Check sheet for the drawn part. Datum: minimum x, y, z corner. Units: mm. A direction names the side the tool comes from. Coordinates: 2 decimals unless noted, no trailing zeros. Write each loop counter-clockwise with the first axis right and the second up, starting at its lowest first coordinate (ties: lowest second). Pieces come first, ordered by that corner, then holes. Notation, with made-up numbers: (-19.5, -20.75) -> (0.5, -20.75) arc R26 cw to (0.5, 15.25) -> close; hole circle Ø2 at (-39, -7.5). An arc over 180 degrees is marked (long way). Answer in a Markdown table with one row per item. Add a question column.
Q1. Thickness scan on line 1 (Z direction, x = 10, y = 63.5); line 2 (Z direction, x = 11, y = 16); line 3 (Y direction, x = 6.25, z = 8). Record the ranges inside material, lowest first.
Q2. Section check A-A, the plane x = 5.5. Record the boundary of the cut face in (y, z).
Q3. Section check C-C, the plane z = 7. Record the boundary of the cut face in (x, y) (1 decimal).
Q4. Section check D-D, the plane x = 1. Record the boundary of the cut face in (y, z), and give its area (3 significant figures).
Q5. Section check B-B, the plane y = 36. Record the boundary of the cut face in (x, z).
Q6. Gauge pin test, flat ends, axial feed: P1, Ø6, axis at x = 8, y = 55, coming from the +Z side; P2, Ø6, axis at x = 7, y = 53, coming from the -Z side; P3, Ø10, axis at y = 65, z = 4, coming from the +X side (3 decimals). Record the tip position at first contact, or that the pin passes through.
Q7. Tool access check on the marked faces 1, 2, 3 and 4. Record the directions out of +Z, -Z, +X, -X, +Y, -Y that give a thin tool (end or side, any length) a straight path to the whole face; none if there is none.
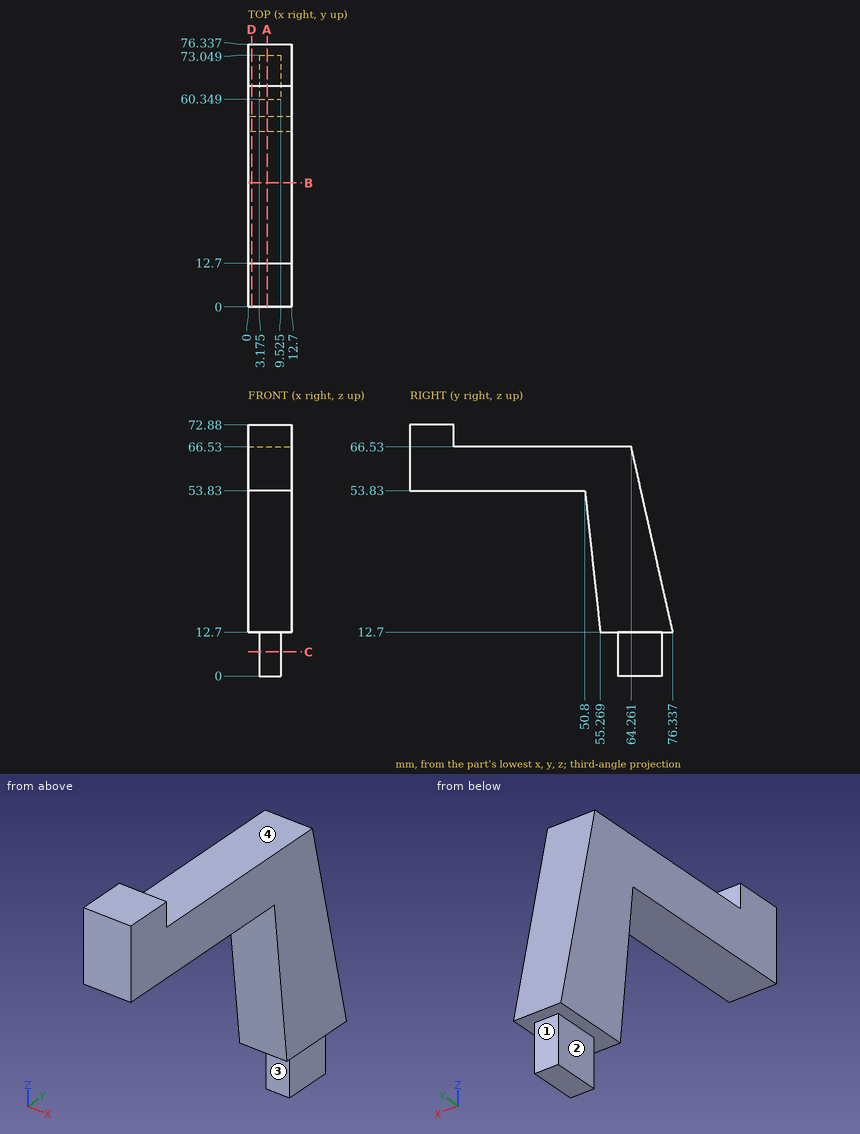
Calculated:
| question | item | result |
|---|---|---|
| 1 | line 1 | z = 12.7 to 66.53 |
| 1 | line 2 | z = 53.83 to 66.53 |
| 1 | line 3 | y = 60.35 to 73.05 |
| 2 | outline | (0, 53.83) -> (50.8, 53.83) -> (55.27, 12.7) -> (60.35, 12.7) -> (60.35, 0) -> (73.05, 0) -> (73.05, 12.7) -> (76.34, 12.7) -> (64.26, 66.53) -> (12.7, 66.53) -> (12.7, 72.88) -> (0, 72.88) -> close |
| 3 | outline | (3.2, 60.3) -> (9.5, 60.3) -> (9.5, 73) -> (3.2, 73) -> close |
| 4 | outline | (0, 53.83) -> (50.8, 53.83) -> (55.27, 12.7) -> (76.34, 12.7) -> (64.26, 66.53) -> (12.7, 66.53) -> (12.7, 72.88) -> (0, 72.88) -> close |
| 4 | area | 1,680 mm² |
| 5 | outline | (0, 53.83) -> (12.7, 53.83) -> (12.7, 66.53) -> (0, 66.53) -> close |
| 6 | P1 | stops at z = 66.53 |
| 6 | P2 | stops at z = 12.7 |
| 6 | P3 | stops at x = 9.525 |
| 7 | face 1 | -Z, +X, -X, +Y |
| 7 | face 2 | -Z, -X, +Y, -Y |
| 7 | face 3 | -Z, +X, -X, -Y |
| 7 | face 4 | +Z, +X, -X, +Y |
